The model under review builds one solid part; all positions refer to its coordinate system, in mm. A direction names the side the tool comes from. Round coordinates to 2 decimals unless told otherwise and drop trailing zeros. Order: outer loops, then holes, each group sorted by start corner. A loop starts at its lowest first (then second) coordinate and runs counter-clockwise, first axis right, second up. Notation, with made-up numbers: M 23,68.25 L 51,68.25 A18 cw 51,85.25 Z; hole C 41,78.5 d3. An arc over 180 degrees is marked long. Answer as a JSON object with one key per item and string values. Group by question number.
1. Add section A-A on z = -1.75. State the section outline as (x, y) points.
2. Clearance check with flat-ended pins moving along their axes: P1, Ø0.5, axis at y = 0.5, z = 6.5, coming from the -X side; P2, Ø1.5, axis at x = 1.5, z = 13, coming from the +Y side; P3, Ø1.5, axis at x = 11.5, z = -4.5, coming from the -Y side; P4, Ø5.5, axis at x = 1.5, z = -11.5, coming from the +Y side. State where each tip first meets the part, or that it passes through.
3. To check wall thickness, follow probe 1 along X at (y, z) = (0.75, 10); probe 2 along Y at (x, z) = (-9.5, -12). State the ranges of each line that lie inside material, in increasing order. Write a range as [from, to].
4. Add section C-C on y = 0.45. State the section outline as (x, z) points.
5. Add section B-B on x = -6.5. State the section outline as (y, z) points, and give its area (3 significant figures).
6. Machinability: for faces 1 (the face through (10, 0.5, -0.2)), 2 (the face through (0.2, 1.5, -10)), 3 (the face through (-10, 0.5, 0.2)), 4 (the face through (-0.2, 1.5, 10)), which of the approach directions +Z, -Z, +X, -X, +Y, -Y give a long, thin tool a straight path to every point of the face, cutting with its end or side? Answer none if there is none.
7. Add section D-D on x = 11.25. State the section outline as (y, z) points, and give its area (3 significant figures).
Autodesk Fusion 360 part; units mm, degrees
sketch "Sketch1" plane through (0, 0, 0) normal (0, 1, 0) x (1, 0, 0)
  line L0 (10, -15) -> (-10, -15)
  line L1 (-10, -15) -> (-10, 15)
  line L2 (-10, 15) -> (10, 15)
  line L3 (10, 15) -> (10, -15)
  line L4 (10, -15) -> (-10, 15) construction
  line L5 (-10, -15) -> (10, 15) construction
  dimension "d1" = 20
  dimension "d2" = 30
extrude "Extrude1" add sketch "Sketch1" along normal blind 1
sketch "Sketch2" plane through (0, 1, 0) normal (0, 1, 0) x (-1, 0, 0)
  line L0 (-10, -15) -> (10, -15)
  line L1 (10, -15) -> (10, 15)
  line L2 (10, 15) -> (-10, 15)
  line L3 (-10, 15) -> (-10, -15)
  line L4 (-10, 10) -> (10, 10)
  line L5 (10, 10) -> (10, -10)
  line L6 (10, -10) -> (-10, -10)
  line L7 (-10, -10) -> (-10, 10)
  line L8 (-10, 10) -> (10, -10) construction
  line L9 (10, 10) -> (-10, -10) construction
  dimension "d5" = 20
extrude "Extrude2" add sketch "Sketch2" along normal blind 0.04 contours L1 L3 L4 L5 L6 L7
sketch "Sketch3" plane through (0, 1.04, 0) normal (0, 1, 0) x (-1, 0, 0)
  line L0 (-10, -10) -> (10, -10)
  line L1 (10, -10) -> (10, 10)
  line L2 (10, 10) -> (-10, 10)
  line L3 (-10, 10) -> (-10, -10)
  line L4 (-15, 10) -> (15, 10)
  line L5 (15, 10) -> (15, -10)
  line L6 (15, -10) -> (-15, -10)
  line L7 (-15, -10) -> (-15, 10)
  line L8 (-15, 10) -> (15, -10) construction
  line L9 (15, 10) -> (-15, -10) construction
  dimension "d8" = 30
  dimension "d9" = 20
extrude "Extrude3" add sketch "Sketch3" along normal blind 1
Recorded:
{
 "1": {"outline": "M -15,1.04 L -10,1.04 L -10,0 L 10,0 L 10,1.04 L 15,1.04 L 15,2.04 L -15,2.04 Z"},
 "2": {"P1": "stops at x = -10", "P2": "stops at y = 1", "P3": "stops at y = 1.04", "P4": "stops at y = 2.04"},
 "3": {"probe 1": "x = [-10, 10]", "probe 2": "y = [0, 1]"},
 "4": {"outline": "M -10,-15 L 10,-15 L 10,15 L -10,15 Z"},
 "5": {"outline": "M 0,-15 L 1,-15 L 1,-10 L 2.04,-10 L 2.04,10 L 1,10 L 1,15 L 0,15 Z", "area": "50.8 mm²"},
 "6": {"face 1": "+Z, -Z, +X, -Y", "face 2": "-Z, +X, -X, +Y", "face 3": "+Z, -Z, -X, -Y", "face 4": "+Z, +X, -X, +Y"},
 "7": {"outline": "M 1.04,-10 L 2.04,-10 L 2.04,10 L 1.04,10 Z", "area": "20.0 mm²"}
}
